```python
from build123d import *

# Parameters (mm, degrees)
SKETCH1_R               = 15
BOSS_EXTRUDE1_DEPTH     = 1
CUT_EXTRUDE1_REACH      = 27.145
CUT_EXTRUDE1_END_RADIUS = 15.25
SKETCH3_R               = 1.375
CIRPATTERN1_COUNT       = 4
CUT_EXTRUDE2_REACH      = 27.645
CUT_EXTRUDE2_END_RADIUS = 15.25
CUT_EXTRUDE2_START      = -0.5
SKETCH8_R               = 2.25
CIRPATTERN2_COUNT       = 4


with BuildPart() as part:
    # Sketch1 → Boss-Extrude1 (new body)
    with BuildSketch(Plane(origin=(0, 0, 0), x_dir=(1, 0, 0), z_dir=(0, 1, 0))):
        with Locations(Location((0, 0, 0), (0, 0, 270))):
            Circle(SKETCH1_R)
    extrude(amount=BOSS_EXTRUDE1_DEPTH)

    # Sketch2 → Revolve1 (revolve)
    with BuildSketch(Plane.XY, mode=Mode.PRIVATE) as revolve1_sk:
        with BuildLine():
            Line((0, 1), (-15, 1))
            ThreePointArc((-15, 1), (-9.762812095, 9.965374514), (0, 13.5))
            Line((0, 13.5), (0, 1))
        make_face()
    revolve(revolve1_sk.sketch.rotate(Axis((0, 1, 0), (0, 1, 0)), 180), axis=Axis((0, 1, 0), (0, 1, 0)))

    # Cut-Extrude1: up to this sphere (the profile starts inside it)
    cut_extrude1_end = Location((0, -1.75, 0)) * Sphere(CUT_EXTRUDE1_END_RADIUS, mode=Mode.PRIVATE)
    # Sketch3 → Cut-Extrude1 (cut, up to the surface)
    with BuildSketch(Plane.XZ, mode=Mode.PRIVATE) as cut_extrude1_sk1:
        with Locations(Location((0, 8, 0), (0, 0, 270))):
            Circle(SKETCH3_R)
    cut_extrude1_tool1 = extrude(cut_extrude1_sk1.sketch, amount=-CUT_EXTRUDE1_REACH, mode=Mode.PRIVATE) & cut_extrude1_end
    cut_extrude1 = cut_extrude1_tool1.solids().sort_by_distance((0, 0, 8))[0]
    add(cut_extrude1, mode=Mode.SUBTRACT)

    # CirPattern1: Cut-Extrude1 ×4 about axis
    cirpattern1_axis = Axis((0, 0, 0), (0, 1, 0))
    for i in range(1, CIRPATTERN1_COUNT):
        add(cut_extrude1.rotate(cirpattern1_axis, i * 360 / CIRPATTERN1_COUNT), mode=Mode.SUBTRACT)

    # Cut-Extrude2: up to this sphere (the profile starts inside it)
    cut_extrude2_end = Location((0, -1.75, 0)) * Sphere(CUT_EXTRUDE2_END_RADIUS, mode=Mode.PRIVATE)
    # Sketch8 → Cut-Extrude2 (cut, up to the surface)
    with BuildSketch(Plane.XZ.offset(CUT_EXTRUDE2_START), mode=Mode.PRIVATE) as cut_extrude2_sk1:
        with Locations(Location((-8, 0, 0), (0, 0, 270))):
            Circle(SKETCH8_R)
    cut_extrude2_tool1 = extrude(cut_extrude2_sk1.sketch, amount=-CUT_EXTRUDE2_REACH, mode=Mode.PRIVATE) & cut_extrude2_end
    cut_extrude2 = cut_extrude2_tool1.solids().sort_by_distance((-8, 0.5, 0))[0]
    add(cut_extrude2, mode=Mode.SUBTRACT)

    # CirPattern2: Cut-Extrude2 ×4 about axis
    cirpattern2_axis = Axis((0, 0, 0), (0, 1, 0))
    for i in range(1, CIRPATTERN2_COUNT):
        add(cut_extrude2.rotate(cirpattern2_axis, i * 360 / CIRPATTERN2_COUNT), mode=Mode.SUBTRACT)


solid = part.part
```
Check sheet for the modelled part. Datum: model origin and axes. Units: mm. A direction names the side the tool comes from. Give positions to 0.01 mm unless a question says otherwise; leave off trailing zeros. Write each loop counter-clockwise with the first axis right and the second up, starting at its lowest first coordinate (ties: lowest second). Pieces come first, ordered by that corner, then holes.
Item 1: Cross-section at B-B (z = -9). Enter the section's corners in (x, y).
Item 2: Cross-section at A-A (x = 0). Enter the section's corners in (y, z) (3 decimals), and give its area (3 significant figures).
Item 3: Access from +Z, -Z, +X, -X, +Y, -Y to the whole of each face (thin tool, end or side, straight path). Record for faces 1 (the face through (9.5, 0.5, 0.5)), 2 (the face through (-0.06, 0.246, -9.374)).
Item 4: Scan lines: L1, parallel to X at y = 6.5, z = 1; L2, parallel to Y at x = 1.5, z = -7; L3, parallel to Z at x = -6.5, y = 2.25. Record each from-to range of solid material in increasing order.
Item 5: Gauge pin test, flat ends, axial feed: pin 1 (3.5 mm diameter, centred on x = -1, z = -7.5, fed in from +Y); pin 2 (2 mm diameter, centred on x = -8, z = 0, fed in from -Y); pin 3 (3 mm diameter, centred on x = 5.5, y = 10.5, fed in from -Z); pin 4 (5 mm diameter, centred on x = 0.5, z = 7.5, fed in from +Y). Record the tip position at first contact, or that the pin passes through.
Item 6: Cross-section at D-D (x = -8). Enter the section's corners in (y, z) (3 decimals), and give its area (3 significant figures).
Item 7: Cross-section at C-C (y = 9). Enter the section's corners in (x, z).
Item 8: Draft check along X on faces 3 (the face through (0.66, 0.493, -14.985)), 4 (the face through (0, 0, 0)), 5 (the face through (0.06, 0.246, 9.374)). Enter one of: released by +X, released by -X, zero draft, split by the parting line, or undercut.
Report:
1. outline: (-12, 0) - (-0.94, 0) - (-0.94, 0.5) - (-2.02, 0.5) - (-2.02, 10.39) arc R12.31 ccw to (-12, 1) - close; (0.94, 0) - (12, 0) - (12, 1) arc R12.31 ccw to (2.02, 10.39) - (2.02, 0.5) - (0.94, 0.5) - close
2. outline: (0, -15) - (1, -15) arc R15.25 ccw to (9.542, -10.25) - (0.5, -10.25) - (0.5, -9.375) - (0, -9.375) - close; (0, -6.625) - (0.5, -6.625) - (0.5, -5.75) - (12.374, -5.75) arc R15.25 ccw to (12.374, 5.75) - (0.5, 5.75) - (0.5, 6.625) - (0, 6.625) - close; (0, 9.375) - (0.5, 9.375) - (0.5, 10.25) - (9.542, 10.25) arc R15.25 ccw to (1, 15) - (0, 15) - close
2. area: 213 mm2
3. face 1: +Y
3. face 2: +Y, -Y
4. L1: x = -12.79 to -10.02, -5.98 to 5.98, 10.02 to 12.79
4. L2: y = 0 to 0.5
4. L3: z = -13.2 to -1.68, 1.68 to 13.2
5. pin 1: stops at y = 12.35
5. pin 2: passes through
5. pin 3: stops at z = -9.5
5. pin 4: stops at y = 12.65
6. outline: (0, -12.689) - (1, -12.689) arc R12.983 ccw to (11.037, -2.25) - (0.5, -2.25) - (0.5, -1.375) - (0, -1.375) - close; (0, 1.375) - (0.5, 1.375) - (0.5, 2.25) - (11.037, 2.25) arc R12.983 ccw to (1, 12.689) - (0, 12.689) - close
6. area: 170 mm2
7. outline: circle Ø21.63 at (0, 0); hole circle Ø4.5 at (-8, 0); hole circle Ø4.5 at (0, -8); hole circle Ø4.5 at (0, 8); hole circle Ø4.5 at (8, 0)
8. face 3: split by the parting line
8. face 4: zero draft
8. face 5: undercut
